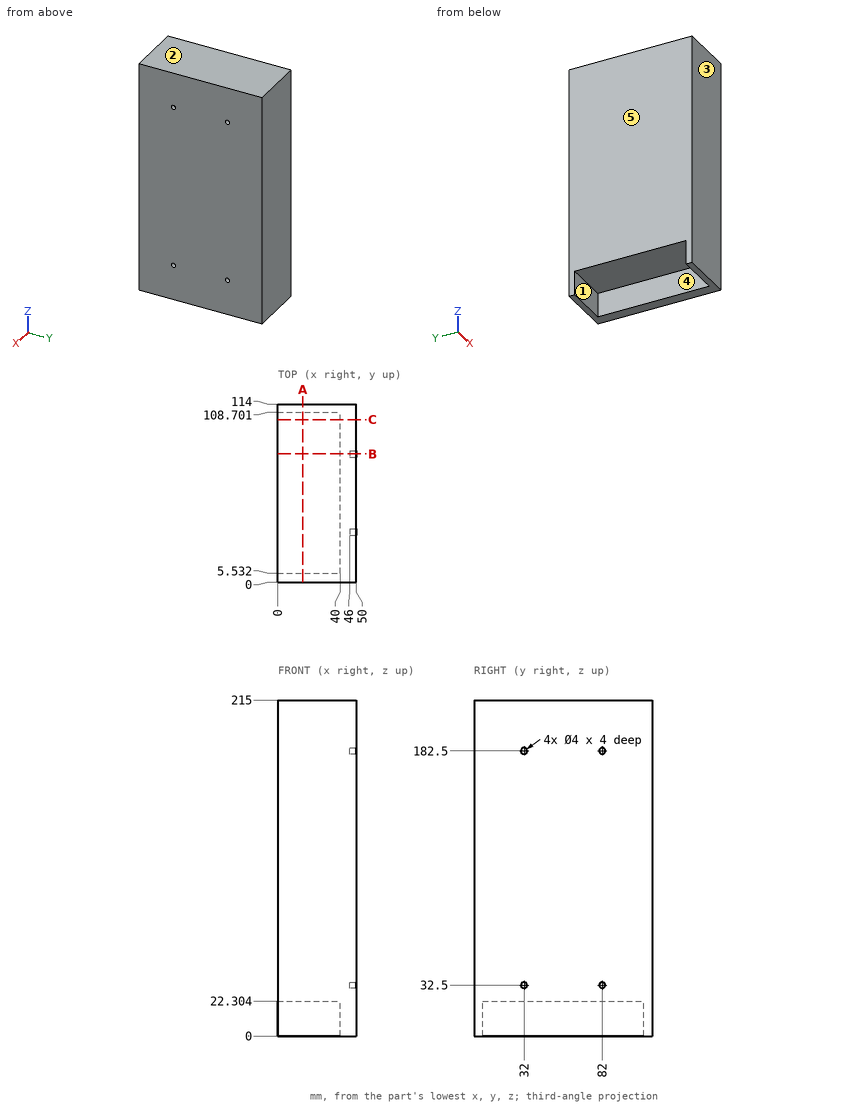
Here's the drawing with two shaded views (mm, measured from the low corner). I have some questions. A direction names the side the tool comes from. Give positions to 0.01 mm unless a question says otherwise; leave off trailing zeros. Order: outer loops, then holes, each group sorted by start corner. A loop starts at its lowest first (then second) coordinate and runs counter-clockwise, first axis right, second up. Notation, with made-up numbers: M 16.25,-13.5 L 45.25,-13.5 A20 cw 45.25,6.5 Z; hole C 68,42 d6. An arc over 180 degrees is marked long. One line per item, written item: value.
1) Please list where these lines run through material, in increasing order: line 1 along Y through (x, z) = (47.45, 32.5); line 2 along Y through (x, z) = (49, 182); line 3 along Y through (x, z) = (33.5, 22).
Answer sheet:
line 1: y = 0 to 30, 34 to 80, 84 to 114
line 2: y = 0 to 30.06, 33.94 to 80.06, 83.94 to 114
line 3: y = 0 to 5.53, 108.7 to 114
2) We'd pull the mould along Y, two halves only. Please class the marked faces 1, 2 and 3: released by +Y, released by -Y, zero draft, split by the parting line, or undercut.
Answer sheet:
face 1: undercut
face 2: zero draft
face 3: released by -Y
3) For P1, Ø3, axis at y = 32, z = 182.5, coming from the +X side, with a flat end and sliding along its axis, tell me the tip position at first contact or that it passes through.
Answer sheet:
P1: stops at x = 46
4) I want a section at C-C, the plane y = 104. List the corners of the cut face in (x, z) for me (1 decimal), plus the area to 3 significant figures.
Answer sheet:
outline: M 0,22.3 L 40,22.3 L 40,0 L 50,0 L 50,215 L 0,215 Z
area: 9,860 mm^2
5) I want a section at B-B, the plane y = 82. List the corners of the cut face in (x, z) for me (1 decimal).
Answer sheet:
outline: M 0,22.3 L 40,22.3 L 40,0 L 50,0 L 50,30.5 L 46,30.5 L 46,34.5 L 50,34.5 L 50,180.5 L 46,180.5 L 46,184.5 L 50,184.5 L 50,215 L 0,215 Z
6) On a 3-axis mill with a long thin cutter (end or side, diameter ignored), from which of +Z, -Z, +X, -X, +Y, -Y can I reach the whole of each face in a straight line? I mean the marked faces 4 and 5. Say none if no direction works.
Answer sheet:
face 4: -Z, -X
face 5: +Z, -Z, -X, +Y, -Y
7) I want a section at A-A, the plane x = 16. List the corners of the cut face in (y, z) for me (1 decimal).
Answer sheet:
outline: M 0,0 L 5.5,0 L 5.5,22.3 L 108.7,22.3 L 108.7,0 L 114,0 L 114,215 L 0,215 Z
